Source: CAD feature listing. Evaluate the final solid. Frame: model axes, mm. A direction names the side the tool comes from. Give positions to 0.01 mm unless a question says otherwise; leave off trailing zeros. Order: outer loops, then holes, each group sorted by start corner. A loop starts at its lowest first (then second) coordinate and runs counter-clockwise, first axis right, second up. Notation, with made-up numbers: M 32.5,-6.75 L 55.5,-6.75 A11 ccw 55.5,-1.75 Z; hole C 65,31.5 d11. An arc over 180 degrees is marked long. Answer as a JSON object with one key per item and string values. Group by question number.
1. Set-up query: faces 1 (the cylindrical face through (68.37, 13.3, 6.26)), 2 (the flat face through (-3, 37.301, 1)). Return all of +Z, -Z, +X, -X, +Y, -Y with unobstructed straight access to the full face (end or side cutting, diameter ignored); none if empty.
2. Section query D-D (y = 40). Output: boundary loops of the cut face in (x, z).
3. Pull-direction query (Y, two-part tool) for faces 3 (the flat face through (8, 14, 2.54)), 4 (the flat face through (-9, -19.382, 6)), 5 (the flat face through (-3, -9.222, 1)), 6 (the flat face through (8, -15, 0)); classes: +Y half, -Y half, draft (parallel to the pull), parting line (faces both ways), or undercut.
4. Section query C-C (z = 10). Output: boundary loops of the cut face in (x, y).
5. Material intervals for L1, parallel to Y at x = 15, z = 1.5; L2, parallel to Z at x = -4.5, y = 28.5; L3, parallel to X at y = 20, z = 2.5, sorted ascending. Write a range as [from, to].
6. Section query B-B (y = 32). Output: boundary loops of the cut face in (x, z), plus the area to 3 significant figures.
7. Section query A-A (x = 29). Output: boundary loops of the cut face in (y, z), plus the area to 3 significant figures.
8. Pin query (flat end, axial travel): P1, Ø5, axis at x = -1, y = -6.5, coming from the -Z side; P2, Ø1.5, axis at y = 16.5, z = 5, coming from the +X side; P3, Ø1.5, axis at x = 42, z = 5, coming from the +Y side. Return the tip coordinate at first contact, or that it passes through.
from build123d import *

# Parameters (mm, degrees)
F0_W     = 85.7403278351
F0_H     = 66.843137145
F1_DEPTH = 12.7
F2_T     = -10.16


with BuildPart() as f1:
    # F0 (on Top) → F1 (new body)
    with BuildSketch(Plane.XY):
        with BuildLine():
            ThreePointArc((34.9580943584, -19.3818807602), (68.379662931, 14.0396878123), (34.9580943584, 47.4612563848))
            Line((34.9580943584, 47.4612563848), (34.9580943584, -19.3818807602))
        make_face()
        with Locations((-7.9120695591, 14.0396878123)):
            Rectangle(F0_W, F0_H)
    extrude(amount=F1_DEPTH)

    # F2
    f2_openings = [f1.faces().sort_by_distance(p)[0] for p in [
        (5.460988, 14.039688, 0),
    ]]
    offset(amount=F2_T, openings=f2_openings)


solid = f1.part
Answer sheet:
{
 "1": {"face 1": "+Z, -Z, +X", "face 2": "-Z"},
 "2": {"outline": "M -50.78,0 L 56.01,0 L 56.01,12.7 L -50.78,12.7 Z"},
 "3": {"face 3": "undercut", "face 4": "-Y half", "face 5": "undercut", "face 6": "draft"},
 "4": {"outline": "M -50.78,-19.38 L 34.96,-19.38 A33.42 ccw 34.96,47.46 L -50.78,47.46 Z"},
 "5": {"L1": "[-19.38, -9.22], [37.3, 47.46]", "L2": "[2.54, 12.7]", "L3": "[-50.78, -40.62], [57.44, 67.84]"},
 "6": {"outline": "M -50.78,0 L -40.62,0 L -40.62,2.54 L 49.74,2.54 L 49.74,0 L 63.14,0 L 63.14,12.7 L -50.78,12.7 Z", "area": "1,220 mm^2"},
 "7": {"outline": "M -19.38,0 L -9.22,0 L -9.22,2.54 L 37.3,2.54 L 37.3,0 L 47.46,0 L 47.46,12.7 L -19.38,12.7 Z", "area": "731 mm^2"},
 "8": {"P1": "z = 2.54", "P2": "x = 68.34", "P3": "y = 46.86"}
}
